The listing builds one solid part. Answer for the finished solid, in the listing's coordinates (mm). Face numbers are marked on the shaded views. A direction names the side the tool comes from. Round coordinates to 2 decimals unless told otherwise and drop trailing zeros. Write each loop counter-clockwise with the first axis right and the second up, starting at its lowest first coordinate (ties: lowest second). Pieces come first, ordered by that corner, then holes.
from build123d import *

# Parameters (mm, degrees)
F0_W     = 8
F0_H     = 7
F0_R     = 0.75
F0_W_2   = 5
F1_DEPTH = 1
F0_W_3   = 1.5
F2_DEPTH = 4
F3_DEPTH = 2.5
F4_W     = 4.784234
F4_H     = 1.5
F5_DEPTH = 5
F6_DEPTH = 2
F7_SIZE  = 0.4


with BuildPart() as f1:
    # F0 (on Top) → F1 (new body)
    with BuildSketch(Plane.XY):
        with Locations((-17.5, 0)):
            Rectangle(F0_W, F0_H)
        Polygon((21.5, 3.5), (21.5, 8.75), (-21.5, 8.75), (-21.5, 3.5), (-13.5, 3.5), (-13.5, -3.5), (-21.5, -3.5), (-21.5, -8.75), (21.5, -8.75), (21.5, -3.5), (16.5, -3.5), (16.5, 3.5), align=None)
        with Locations((-20.3, -7.55)):
            Circle(F0_R, mode=Mode.SUBTRACT)
        with Locations((20.3, -7.55)):
            Circle(F0_R, mode=Mode.SUBTRACT)
        with Locations((-20.3, 7.55)):
            Circle(F0_R, mode=Mode.SUBTRACT)
        with Locations((20.3, 7.55)):
            Circle(F0_R, mode=Mode.SUBTRACT)
        with Locations((19, 0)):
            Rectangle(F0_W_2, F0_H)
    extrude(amount=-F1_DEPTH)

    # F0 (on Top) → F2 (join)
    with BuildSketch(Plane.XY):
        with Locations((-22.25, 0)):
            Rectangle(F0_W_3, F0_H)
        with Locations((-17.5, 0)):
            Rectangle(F0_W, F0_H)
    extrude(amount=F2_DEPTH)

    # F0 (on Top) → F3 (join)
    with BuildSketch(Plane.XY):
        with Locations((19, 0)):
            Rectangle(F0_W_2, F0_H)
    extrude(amount=F3_DEPTH)

    # F4 (on face) → F5 (cut)
    with BuildSketch(Plane(origin=(-23, 0, 0), x_dir=(0, -1, 0), z_dir=(-1, 0, 0))):
        Polygon((3.4, 3.9), (-3.4, 3.9), (-3.4, 2.041421), (-2.9, 1.541421), (-2.9, 0.1), (2.9, 0.1), (2.9, 1.541421), (3.4, 2.041421), align=None)
        with Locations((0, 2.25)):
            Rectangle(F4_W, F4_H, mode=Mode.SUBTRACT)
    extrude(amount=-F5_DEPTH, mode=Mode.SUBTRACT)

    # F4 (on face) → F6 (cut)
    with BuildSketch(Plane(origin=(-23, 0, 0), x_dir=(0, -1, 0), z_dir=(-1, 0, 0))):
        Polygon((-3, 1.5), (-3.5, 2), (-3.5, 0), (-3, 0), align=None)
        Polygon((3, 1.5), (3, 0), (3.5, 0), (3.5, 2), align=None)
    extrude(amount=-F6_DEPTH, mode=Mode.SUBTRACT)

    # F7
    f7_edges = [f1.edges().sort_by_distance(p)[0] for p in [
        (-20.5, -2.392117, 1.5),
        (-20.5, 2.392117, 1.5),
    ]]
    chamfer(f7_edges, length=F7_SIZE)


solid = f1.part
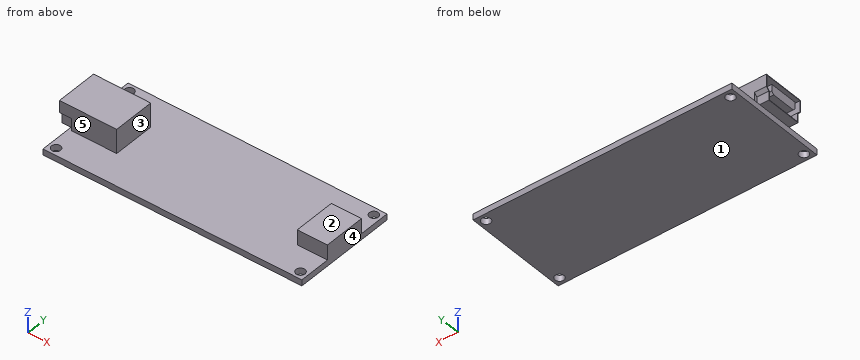
1. Straight lines are drawn through the part: line 1 along Y through (x, z) = (-20.3, -0.15); line 2 along X through (y, z) = (0.75, 0.15); line 3 along Z through (x, y) = (-17, -4.5). For each, find the intervals that lie inside material, in ascending order.
Geometry says:
line 1: y = -8.75 to -8.3, -6.8 to 6.8, 8.3 to 8.75
line 2: x = -18 to -13.5, 16.5 to 21.5
line 3: z = -1 to 0
2. A tool of negligible diameter and unlimited length cuts with its end or side. For the marked faces 1 and 2, from which of +Z, -Z, +X, -X, +Y, -Y can it reach the whole face along a straight path? Write none if from no direction.
Geometry says:
face 1: -Z, +X, -X, +Y, -Y
face 2: +Z, +X, +Y, -Y
3. Section B-B on y = 7.55 is taken. Determine the outline of the cut face in (x, z).
Geometry says:
outline: (-21.5, -1) - (-21.05, -1) - (-21.05, 0) - (-21.5, 0) - close; (-19.55, -1) - (19.55, -1) - (19.55, 0) - (-19.55, 0) - close; (21.05, -1) - (21.5, -1) - (21.5, 0) - (21.05, 0) - close
4. Section D-D on y = 0.75 is taken. Determine the outline of the cut face in (x, z), plus the area to 3 significant figures.
Geometry says:
outline: (-23, 0) - (-21.5, 0) - (-21.5, -1) - (21.5, -1) - (21.5, 2.5) - (16.5, 2.5) - (16.5, 0) - (-13.5, 0) - (-13.5, 4) - (-23, 4) - (-23, 3.9) - (-18, 3.9) - (-18, 3) - (-23, 3) - (-23, 1.5) - (-18, 1.5) - (-18, 0.1) - (-23, 0.1) - close
area: 82.0 mm2
5. Given pin 1 (0.9 mm diameter, centred on x = -20, z = 2.5, fed in from -Y); pin 2 (0.8 mm diameter, centred on x = -22.5, y = 0, fed in from -Z); pin 3 (0.7 mm diameter, centred on x = -20.5, z = 0.5, fed in from +Y), each flat-ended and moving along its own axis, determine where each tip first touches the part or whether it passes through.
Geometry says:
pin 1: stops at y = -3.5
pin 2: stops at z = 0
pin 3: stops at y = 3.5
6. For a pull along X with two mould halves and no side action, classify the marked faces 3, 4 and 5 as released by +X, released by -X, zero draft, split by the parting line, or undercut.
Geometry says:
face 3: undercut
face 4: released by +X
face 5: zero draft
7. Section C-C on x = 20.3 is taken. Determine the outline of the cut face in (y, z), plus the area to 3 significant figures.
Geometry says:
outline: (-8.75, -1) - (-8.3, -1) - (-8.3, 0) - (-8.75, 0) - close; (-6.8, -1) - (6.8, -1) - (6.8, 0) - (3.5, 0) - (3.5, 2.5) - (-3.5, 2.5) - (-3.5, 0) - (-6.8, 0) - close; (8.3, -1) - (8.75, -1) - (8.75, 0) - (8.3, 0) - close
area: 32.0 mm2
8. Section A-A on x = -20.3 is taken. Give the number of separate pieces and of enclosed holes in the cut face, plus the area to 3 significant figures.
Geometry says:
separate pieces: 4
enclosed holes: 1
area: 25.4 mm2
